```python
from build123d import *

# Parameters (mm, degrees)
SKETCH1_R               = 5
BOSS_EXTRUDE1_DEPTH     = 60.8
SKETCH2_R               = 1
CUT_EXTRUDE1_DEPTH      = 6
CUT_EXTRUDE1_DEPTH_BACK = 6
SKETCH3_OUTSIDE_W       = 24.484
SKETCH3_OUTSIDE_H       = 24.484
SKETCH3_OUTSIDE_R       = 3.5
CUT_EXTRUDE2_DEPTH      = 10


with BuildPart() as part:
    # Sketch1 → Boss-Extrude1 (new body)
    with BuildSketch(Plane.XY):
        Circle(SKETCH1_R)
    extrude(amount=BOSS_EXTRUDE1_DEPTH)

    # Sketch2 → Cut-Extrude1 (cut, two sides)
    with BuildSketch(Plane(origin=(0, 0, 0), x_dir=(0, 0, -1), z_dir=(1, 0, 0))) as cut_extrude1_sk:
        with Locations((-2.031417136, 0)):
            Circle(SKETCH2_R)
    extrude(amount=CUT_EXTRUDE1_DEPTH, mode=Mode.SUBTRACT)
    extrude(cut_extrude1_sk.sketch, amount=-CUT_EXTRUDE1_DEPTH_BACK, mode=Mode.SUBTRACT)

    # Sketch3 outside → Cut-Extrude2 (cut)
    with BuildSketch(Plane(origin=(0, 0, 0), x_dir=(-1, 0, 0), z_dir=(0, 0, -1))):
        Rectangle(SKETCH3_OUTSIDE_W, SKETCH3_OUTSIDE_H)
        Circle(SKETCH3_OUTSIDE_R, mode=Mode.SUBTRACT)
    extrude(amount=-CUT_EXTRUDE2_DEPTH, mode=Mode.SUBTRACT)


solid = part.part
```
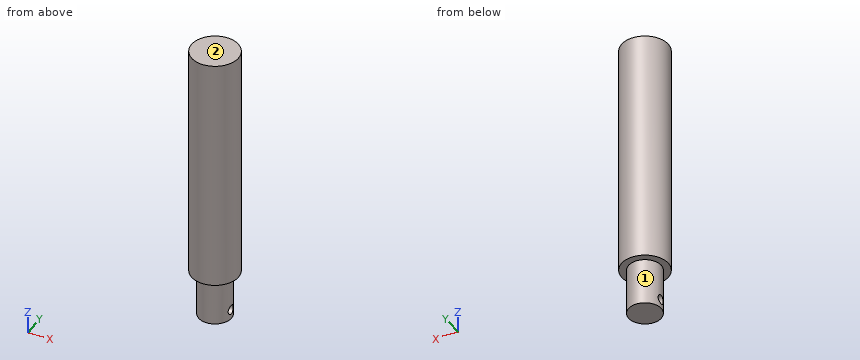
Here's how the part is built. I have some questions about the finished solid (model axes, mm). Face numbers are marked on the shaded views. A direction names the side the tool comes from. Coordinates: 2 decimals unless noted, no trailing zeros. Order: outer loops, then holes, each group sorted by start corner. A loop starts at its lowest first (then second) coordinate and runs counter-clockwise, first axis right, second up. Notation, with made-up numbers: M 83.5,13 L 125.5,13 A32 ccw 125.5,43 Z; hole C 19.5,86 d7. An arc over 180 degrees is marked long. Answer as a JSON object with one key per item and string values. Group by question number.
(1) Which directions (+Z, -Z, +X, -X, +Y, -Y) give clear straight access to the entire face, cutting with the end or side of a thin tool? Please do the marked faces 1 and 2.
(2) For pin 1 (5 mm diameter, centred on x = -0.5, z = 35, fed in from +Y); pin 2 (1.5 mm diameter, centred on y = -4, z = 11, fed in from -X), each with a flat end and sliding along its axis, tell me the tip position at first contact or that it passes through.
(3) Suppose I cut it at B-B, the plane x = 0. Please give me the cut outline in (y, z), then the cut area to 3 significant figures.
(4) Suppose I cut it at C-C, the plane z = 26.5. Please give me the cut outline in (x, y).
(5) Suppose I cut it at D-D, the plane y = 2.75. Please give me the cut outline in (x, z).
(6) I need wall thicknesses on probe 1 along Z at (x, y) = (-1.5, 0); probe 2 along Y at (x, z) = (0.25, 42); probe 3 along Z at (x, y) = (0, -3.75). Which ranges of each line are inside material? Lowest first, please.
(7) Suppose I cut it at A-A, the plane y = 0. Please give me the cut outline in (x, z).
Values found:
{
 "1": {"face 1": "-Z", "face 2": "+Z, +X, -X, +Y, -Y"},
 "2": {"pin 1": "stops at y = 5", "pin 2": "stops at x = -3.8"},
 "3": {"outline": "M -5,10 L -3.5,10 L -3.5,0 L 3.5,0 L 3.5,10 L 5,10 L 5,60.8 L -5,60.8 Z; hole C 0,2.03 d2", "area": "575 mm^2"},
 "4": {"outline": "C 0,0 d10"},
 "5": {"outline": "M -4.18,10 L -2.17,10 L -2.17,0 L 2.17,0 L 2.17,10 L 4.18,10 L 4.18,60.8 L -4.18,60.8 Z"},
 "6": {"probe 1": "z = 0 to 1.03, 3.03 to 60.8", "probe 2": "y = -4.99 to 4.99", "probe 3": "z = 10 to 60.8"},
 "7": {"outline": "M -5,10 L -3.5,10 L -3.5,3.03 L 3.5,3.03 L 3.5,10 L 5,10 L 5,60.8 L -5,60.8 Z; M -3.5,0 L 3.5,0 L 3.5,1.03 L -3.5,1.03 Z"}
}
